Part model, mm, in its own coordinate system. A direction names the side the tool comes from. Round coordinates to 2 decimals unless told otherwise and drop trailing zeros. Loops run counter-clockwise (first coordinate to the right, second up) from the corner with the lowest first, then second, coordinate; pieces in that order, holes last. Notation, with made-up numbers: (-5, -29) - (31, -29) arc R30 ccw to (31, -5) - close; hole circle Ø8 at (-24, 20). An arc over 180 degrees is marked (long way). Write each question's results on one line, items separated by ' | '. Start each with the question number.
(1) Cut at D-D, the plane z = -39. List the corners of the cut face in (x, y), then the cut area to 3 significant figures.
(2) Mould opens along Y. For faces 5 (the face through (20, -4, -87)), 6 (the face through (-93.77, -63.99, -146.96)), 7 (the face through (-5, -6, -51)), 8 (the face through (27, -235, -147)) say: released by +Y, released by -Y, zero draft, split by the parting line, or undercut.
(3) Drill centre lines: L1, parallel to Z at x = -49, y = -198; L2, parallel to Z at x = 105, y = -212.5; L3, parallel to Y at x = -24.5, z = -94. Where is each one in solid material? Low to high.
(4) Tool access for faces 1 (the face through (31, -252, -147)), 2 (the face through (-7, -158, -144)), 3 (the face through (-10.72, -304.74, -146.96)), 4 (the face through (85.82, -64.24, -146.96)): list every direction of +Z, -Z, +X, -X, +Y, -Y with a clear straight run to the whole face (end or side of a thin tool).
(5) Flat gauge pin, fed straight in: P1, Ø3, axis at x = 1, y = -141.5, coming from the +Z side. Where does the tip first touch, or does it go through?
(6) Cut at C-C, the plane y = -130. List the corners of the cut face in (x, z).
(7) Cut at B-B, the plane y = -51. List the corners of the cut face in (x, z).
(8) Cut at A-A, the plane x = -131. List the corners of the cut face in (y, z), then the cut area to 3 significant figures.
from build123d import *

# Parameters (mm, degrees)
F0_W     = 50
F0_H     = 6
F2_DEPTH = 130
F0_H_2   = 100
F0_H_3   = 74
F3_DEPTH = 6
F4_R     = 20
F5_R     = 10
F7_DEPTH = 6
F9_DEPTH = 3


with BuildPart() as f2:
    # F0 (on Front) → F2 (new body)
    with BuildSketch(Plane.XZ):
        with Locations((-5, -147)):
            Rectangle(F0_W, F0_H)
    extrude(amount=F2_DEPTH)

    # F0 (on Front) → F3 (join)
    with BuildSketch(Plane.XZ):
        with Locations((-5, -20)):
            Rectangle(F0_W, F0_H_2)
        with Locations((-5, -107)):
            Rectangle(F0_W, F0_H_3)
        with Locations((-5, -147)):
            Rectangle(F0_W, F0_H)
    extrude(amount=F3_DEPTH)

    # F4
    f4_edges = [f2.edges().sort_by_distance(p)[0] for p in [
        (-5, 0, -150),
    ]]
    fillet(f4_edges, radius=F4_R)

    # F5
    f5_edges = [f2.edges().sort_by_distance(p)[0] for p in [
        (-5, -6, -144),
    ]]
    fillet(f5_edges, radius=F5_R)

    # F6 (on face) → F7 (join)
    with BuildSketch(Plane.XY.offset(-144)):
        with BuildLine():
            ThreePointArc((-30, -73.708494), (-94.658376, -63.779027), (-156.74109, -43.162615))
            ThreePointArc((-156.74109, -43.162615), (-5.609318, -304.830543), (147.342686, -44.222404))
            ThreePointArc((147.342686, -44.222404), (84.92667, -64.450181), (20, -73.90796))
            Line((20, -73.90796), (20, -130))
            Line((20, -130), (-30, -130))
            Line((-30, -130), (-30, -73.708494))
        make_face()
    extrude(amount=-F7_DEPTH)

    # F8 (on face) → F9 (cut)
    with BuildSketch(Plane.XY.offset(-144)):
        with BuildLine():
            ThreePointArc((-5, -254.552964), (-127.681443, -193.636873), (-153.304019, -59.082088))
            Line((-153.304019, -59.082088), (-162.379453, -55.630867))
            ThreePointArc((-162.379453, -55.630867), (-135.651994, -199.132241), (-5, -264.224927))
            ThreePointArc((-5, -264.224927), (125.651994, -199.132241), (152.379453, -55.630867))
            Line((152.379453, -55.630867), (143.304019, -59.082088))
            ThreePointArc((143.304019, -59.082088), (117.681443, -193.636873), (-5, -254.552964))
        make_face()
        with BuildLine():
            Line((-136.756967, -65.374629), (-144.992024, -62.242987))
            ThreePointArc((-144.992024, -62.242987), (-120.384014, -188.605777), (-5, -245.699019))
            ThreePointArc((-5, -245.699019), (110.384014, -188.605777), (134.992024, -62.242987))
            Line((134.992024, -62.242987), (126.756967, -65.374629))
            ThreePointArc((126.756967, -65.374629), (103.157098, -183.623516), (-5, -236.932005))
            ThreePointArc((-5, -236.932005), (-113.157098, -183.623516), (-136.756967, -65.374629))
        make_face()
    extrude(amount=-F9_DEPTH, mode=Mode.SUBTRACT)


solid = f2.part
A:
1) outline: (-30, -6) - (20, -6) - (20, 0) - (-30, 0) - close | area: 300 mm2
2) face 5: zero draft | face 6: released by +Y | face 7: released by -Y | face 8: undercut
3) L1: -150 to -144 | L2: -150 to -147 | L3: -6 to 0
4) face 1: +Z | face 2: +Z, +X, -X, -Y | face 3: +Z, -Z | face 4: +Z, -Z, +Y
5) P1: z = -144
6) outline: (-179.83, -150) - (169.83, -150) - (169.83, -144) - (156, -144) - (156, -147) - (146.15, -147) - (146.15, -144) - (137.12, -144) - (137.12, -147) - (128.16, -147) - (128.16, -144) - (-138.16, -144) - (-138.16, -147) - (-147.12, -147) - (-147.12, -144) - (-156.15, -144) - (-156.15, -147) - (-166, -147) - (-166, -144) - (-179.83, -144) - close
7) outline: (-160.97, -150) - (-136.97, -150) - (-136.97, -144) - (-160.97, -144) - close; (-30, -150) - (20, -150) - (20, -144) - (-30, -144) - close; (130.07, -150) - (150.97, -150) - (150.97, -144) - (130.07, -144) - close
8) outline: (-251.2, -150) - (-53.13, -150) - (-53.13, -144) - (-152.73, -144) - (-152.73, -147) - (-172.6, -147) - (-172.6, -144) - (-189.09, -144) - (-189.09, -147) - (-205.01, -147) - (-205.01, -144) - (-251.2, -144) - close | area: 1,080 mm2
